Source: CAD feature listing. Evaluate the final solid. Frame: model axes, mm. Give positions to 0.01 mm unless a question says otherwise; leave off trailing zeros. Loops run counter-clockwise (first coordinate to the right, second up) from the corner with the lowest first, then second, coordinate; pieces in that order, holes last.
```python
from build123d import *

# Parameters (mm, degrees)
F1_DEPTH = 1.5
F3_DEPTH = 3.001
F4_R     = 1
F7_W     = 1
F7_H     = 4.0566037736
F8_DEPTH = 3.5


# Not quite as in the source:
# - a feature names something its author has since deleted; it is built from what else it names


with BuildPart() as f1:
    # F0 (on Top) → F1 (new body, symmetric)
    with BuildSketch(Plane.XY):
        Polygon((0, 1.5), (-26.5, 8.5), (-26.5, 0), (-26.5, -8.5), (0, -1.5), (26.5, -8.5), (26.5, 0), (26.5, 8.5), align=None)
    extrude(amount=F1_DEPTH, both=True)

    # F2 (on face) → F3 (cut, through all)
    with BuildSketch(Plane.XY.offset(1.5)):
        Polygon((-24.5, 5.9030988568), (-24.5, 0), (-24.5, -5.9030988568), (-2.1525543278, 0), align=None)
        Polygon((24.5, 0), (24.5, 5.9030988568), (2.1525543278, 0), (24.5, -5.9030988568), align=None)
    extrude(amount=-F3_DEPTH, mode=Mode.SUBTRACT)

    # F4
    f4_edges = [f1.edges().sort_by_distance(p)[0] for p in [
        (-2.152554, 0, 0),
        (2.152554, 0, 0),
    ]]
    fillet(f4_edges, radius=F4_R)

    # F5 (on Top) → F6 (revolve)
    with BuildSketch(Plane.XY):
        Polygon((20.5, 8.5), (35.5, 8.5), (35.5, 10), (33.5, 10), (33.5, 10.5), (32.5, 10.5), (32.5, 10), (29.5, 10), (29.5, 10.5), (28.5, 10.5), (28.5, 10), (20.5, 10), align=None)
    revolve(axis=Axis((28, 8.5, 0), (1, 0, 0)))

    # F7 (on Top) → F8 (join, symmetric)
    with BuildSketch(Plane.XY):
        with Locations((-2.5, 0)):
            Rectangle(F7_W, F7_H)
    extrude(amount=F8_DEPTH, both=True)

    # F9: F1 across plane


with BuildPart() as f1_1:
    add(f1.part)
    add(f1.part.mirror(Plane.YZ))

    # F10: F1 across plane


with BuildPart() as f1_2:
    add(f1_1.part)
    add(f1_1.part.mirror(Plane.XZ))


solid = f1_2.part
```
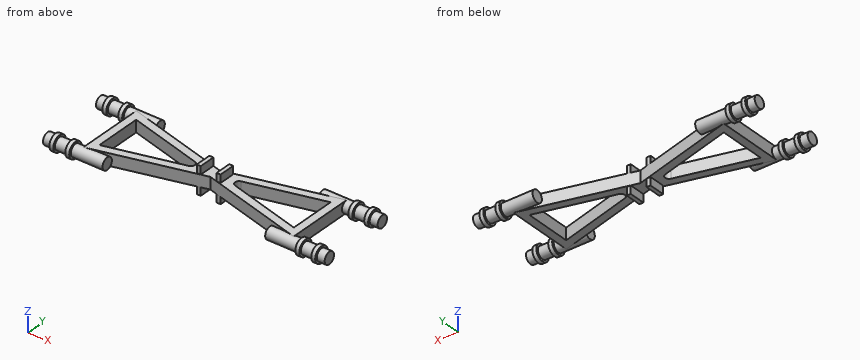
(1) Section C-C, the plane z = 0. Count the separate pieces of the cut face and the enclosed holes in it, then the cut area to 3 significant figures.
A:
separate pieces: 1
enclosed holes: 2
area: 442 mm2
(2) Section D-D, the plane x = 31. Return the cut outline in (y, z), then the cut area to 3 significant figures.
A:
outline: circle Ø3 at (-8.5, 0); circle Ø3 at (8.5, 0)
area: 14.1 mm2
(3) Ray query, line 1 along X through (y, z) = (9.25, 0.5); line 2 along X through (y, z) = (1.75, 3.25); line 3 along Z through (x, y) = (-19, 6). Return the intervals inside material, ascending.
A:
line 1: x = -35.5 to -20.5, 20.5 to 35.5
line 2: x = -3 to -2, 2 to 3
line 3: z = -1.5 to 1.5
(4) Section B-B, the plane x = 9.5. Return the cut outline in (y, z), then the cut area to 3 significant figures.
A:
outline: (-4.01, -1.5) - (-1.94, -1.5) - (-1.94, 1.5) - (-4.01, 1.5) - close; (1.94, -1.5) - (4.01, -1.5) - (4.01, 1.5) - (1.94, 1.5) - close
area: 12.4 mm2
(5) First-contact query: pin 1 (0.9 mm diameter, centred on y = -2.5, z = -0.5, fed in from -X); pin 2 (0.6 mm diameter, centred on y = 0, z = -2.5, fed in from +X); pin 3 (1 mm diameter, centred on y = -0.5, z = -2.5, fed in from -X). Flat tips, straight axial feed; report the tip coordinate or a pass-through.
A:
pin 1: stops at x = -26.5
pin 2: stops at x = 3
pin 3: stops at x = -3
(6) Section A-A, the plane y = 3.75. Return the cut outline in (x, z).
A:
outline: (-26.5, -1.5) - (-24.5, -1.5) - (-24.5, 1.5) - (-26.5, 1.5) - close; (-16.35, -1.5) - (-8.52, -1.5) - (-8.52, 1.5) - (-16.35, 1.5) - close; (8.52, -1.5) - (16.35, -1.5) - (16.35, 1.5) - (8.52, 1.5) - close; (24.5, -1.5) - (26.5, -1.5) - (26.5, 1.5) - (24.5, 1.5) - close
